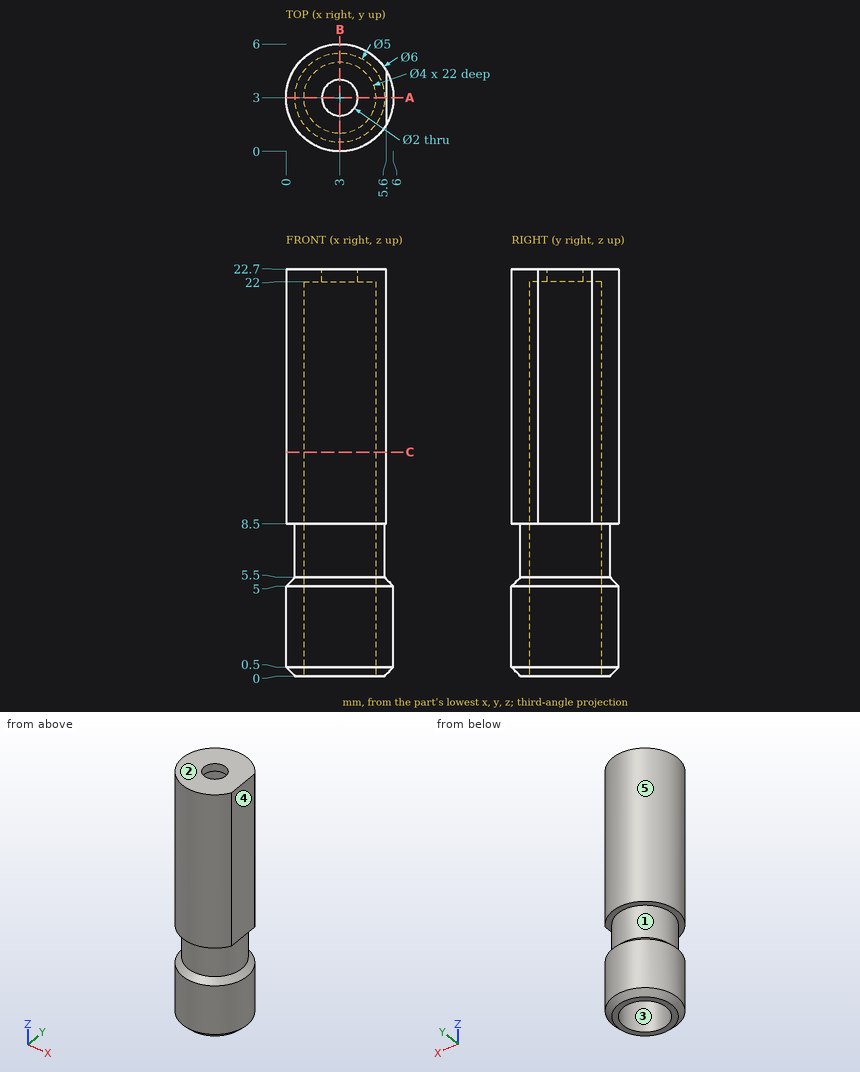
Geometry check sheet. Reference: drawing and pictorial views, mm from the part's lowest x, y, z. A direction names the side the tool comes from. Give positions to 0.01 mm unless a question says otherwise; leave off trailing zeros. Order: outer loops, then holes, each group sorted by start corner. A loop starts at its lowest first (then second) coordinate and runs counter-clockwise, first axis right, second up. Notation, with made-up numbers: (17.25, -39.5) - (25.25, -39.5) arc R32 ccw to (25.25, -12.5) - close; hole circle Ø7 at (-38.75, 23.5). An arc over 180 degrees is marked (long way). Answer as CSV lines item,"result". Start each with the question number.
Item 1: Access from +Z, -Z, +X, -X, +Y, -Y to the whole of each face (thin tool, end or side, straight path). Record for the marked faces 1 and 2.
Item 2: Section check A-A, the plane y = 3. Record the boundary of the cut face in (x, z), plus the area to 3 significant figures.
Item 3: Section check C-C, the plane z = 12.5. Record the boundary of the cut face in (x, y), plus the area to 3 significant figures.
Item 4: Gauge pin test, flat ends, axial feed: pin 1 (1.7 mm diameter, centred on x = 4, y = 1.5, fed in from -Z); pin 2 (1 mm diameter, centred on x = 2, z = 12.5, fed in from -Y); pin 3 (3.5 mm diameter, centred on y = 2.5, z = 16.5, fed in from +X); pin 4 (3 mm diameter, centred on x = 3, y = 3, fed in from -Z). Record the tip position at first contact, or that the pin passes through.
Item 5: Mould release check, pull along Y, two halves, no side actions. Record for the marked faces 3, 4 and 5: released by +Y, released by -Y, zero draft, split by the parting line, or undercut.
Item 6: Material ranges on L1, parallel to Y at x = 3, z = 22.25; L2, parallel to Y at x = 3, z = 12; L3, parallel to Z at x = 2.1, y = 4.75, recorded low to high.
Item 7: Section check B-B, the plane x = 3. Record the boundary of the cut face in (y, z).
Filled in:
1,face 1,"none"
1,face 2,"+Z, +X, -X, +Y, -Y"
2,outline,"(0, 0.5) - (0.5, 0) - (1, 0) - (1, 22) - (2, 22) - (2, 22.7) - (0, 22.7) - (0, 8.5) - (0.5, 8.5) - (0.5, 5.5) - (0, 5) - close; (4, 22) - (5, 22) - (5, 0) - (5.5, 0) - (6, 0.5) - (6, 5) - (5.5, 5.5) - (5.5, 8.5) - (5.6, 8.5) - (5.6, 22.7) - (4, 22.7) - close"
2,area,"37.6 mm^2"
3,outline,"(5.6, 1.5) - (5.6, 4.5) arc R3 ccw (long way) to start; hole circle Ø4 at (3, 3)"
3,area,"14.9 mm^2"
4,pin 1,"z = 0"
4,pin 2,"y = 0.04"
4,pin 3,"x = 5.6"
4,pin 4,"z = 22"
5,face 3,"undercut"
5,face 4,"zero draft"
5,face 5,"split by the parting line"
6,L1,"0 to 2, 4 to 6"
6,L2,"0 to 1, 5 to 6"
6,L3,"22 to 22.7"
7,outline,"(0, 0.5) - (0.5, 0) - (1, 0) - (1, 22) - (2, 22) - (2, 22.7) - (0, 22.7) - (0, 8.5) - (0.5, 8.5) - (0.5, 5.5) - (0, 5) - close; (4, 22) - (5, 22) - (5, 0) - (5.5, 0) - (6, 0.5) - (6, 5) - (5.5, 5.5) - (5.5, 8.5) - (6, 8.5) - (6, 22.7) - (4, 22.7) - close"
